from build123d import *

# Parameters (mm, degrees)
SKETCH1_W             = 15
SKETCH1_H             = 21.5
BOSS_EXTRUDE1_DEPTH   = 2.5
CHAMFER1_SIZE         = 1.5
CHAMFER1_SIZE2        = 1.7
CHAMFER1_PART_2_SIZE  = 1.5
CHAMFER1_PART_2_SIZE2 = 1.7
CHAMFER1_PART_3_SIZE  = 1.5
CHAMFER1_PART_3_SIZE2 = 1.7
CHAMFER1_PART_4_SIZE  = 1.5
CHAMFER1_PART_4_SIZE2 = 1.7
SKETCH3_W             = 11.7
SKETCH3_H             = 18
BOSS_EXTRUDE2_DEPTH   = 11
SKETCH4_W             = 6.25827791
SKETCH4_H             = 0.502489468
SKETCH4_H_2           = 0.571010759
SKETCH4_H_3           = 0.593851189
BOSS_EXTRUDE3_DEPTH   = 7
SKETCH5_R             = 0.857772401
CUT_EXTRUDE1_DEPTH    = 22
BOSS_EXTRUDE4_DEPTH   = 22
SKETCH8_W             = 6.303958771
SKETCH8_H             = 16.703004391
SKETCH8_W_2           = 12.882002706
SKETCH8_H_2           = 17.251174719
CUT_EXTRUDE2_DEPTH    = 16


with BuildPart() as part:
    # Sketch1 → Boss-Extrude1 (new body)
    with BuildSketch(Plane(origin=(0, 0, 0), x_dir=(1, 0, 0), z_dir=(0, 1, 0))):
        with Locations((1.401590457, -5.203280318)):
            Rectangle(SKETCH1_W, SKETCH1_H)
    extrude(amount=BOSS_EXTRUDE1_DEPTH)

    # Chamfer1
    chamfer1_edges = [part.edges().sort_by_distance(p)[0] for p in [
        (8.901590457, 2.5, 5.203280318),
    ]]
    chamfer1_side = [part.faces().sort_by_distance(p)[0] for p in [
        (8.901590457, 1.25, 5.203280318),
    ]]
    chamfer(chamfer1_edges, length=CHAMFER1_SIZE, length2=CHAMFER1_SIZE2, reference=chamfer1_side[0])

    # Chamfer1 part 2
    chamfer1_part_2_edges = [part.edges().sort_by_distance(p)[0] for p in [
        (1.401590457, 2.5, -5.546719682),
    ]]
    chamfer1_part_2_side = [part.faces().sort_by_distance(p)[0] for p in [
        (1.401590457, 1.25, -5.546719682),
    ]]
    chamfer(chamfer1_part_2_edges, length=CHAMFER1_PART_2_SIZE, length2=CHAMFER1_PART_2_SIZE2, reference=chamfer1_part_2_side[0])

    # Chamfer1 part 3
    chamfer1_part_3_edges = [part.edges().sort_by_distance(p)[0] for p in [
        (-6.098409543, 2.5, 5.203280318),
    ]]
    chamfer1_part_3_side = [part.faces().sort_by_distance(p)[0] for p in [
        (-6.098409543, 1.25, 5.203280318),
    ]]
    chamfer(chamfer1_part_3_edges, length=CHAMFER1_PART_3_SIZE, length2=CHAMFER1_PART_3_SIZE2, reference=chamfer1_part_3_side[0])

    # Chamfer1 part 4
    chamfer1_part_4_edges = [part.edges().sort_by_distance(p)[0] for p in [
        (1.401590457, 2.5, 15.953280318),
    ]]
    chamfer1_part_4_side = [part.faces().sort_by_distance(p)[0] for p in [
        (1.401590457, 1.25, 15.953280318),
    ]]
    chamfer(chamfer1_part_4_edges, length=CHAMFER1_PART_4_SIZE, length2=CHAMFER1_PART_4_SIZE2, reference=chamfer1_part_4_side[0])

    # Sketch3 → Boss-Extrude2 (add)
    with BuildSketch(Plane.XZ):
        with Locations((1.324498787, 5.226991199)):
            Rectangle(SKETCH3_W, SKETCH3_H)
    extrude(amount=BOSS_EXTRUDE2_DEPTH)

    # Sketch4 → Boss-Extrude3 (add)
    with BuildSketch(Plane.XZ.offset(11)):
        with Locations((1.23028723, 12.923345769)):
            Rectangle(SKETCH4_W, SKETCH4_H)
        with Locations((1.23028723, 5.854232582)):
            Rectangle(SKETCH4_W, SKETCH4_H_2)
        with Locations((1.23028723, -2.265540399)):
            Rectangle(SKETCH4_W, SKETCH4_H_3)
    extrude(amount=BOSS_EXTRUDE3_DEPTH)

    # Sketch5 → Cut-Extrude1 (cut)
    with BuildSketch(Plane(origin=(0, 0, -2.562465994), x_dir=(-1, 0, 0), z_dir=(0, 0, -1))):
        with Locations((-1.203624554, -14.610197603)):
            Circle(SKETCH5_R)
        Polygon((-3.009226286, -18.607426263), (-4.889542572, -15.232818889), (-5.175948364, -18.482902006), align=None)
        Polygon((0.726501434, -18.545164135), (2.357769206, -15.232818889), (2.818508958, -18.545164135), align=None)
    extrude(amount=-CUT_EXTRUDE1_DEPTH, mode=Mode.SUBTRACT)

    # Sketch7 → Boss-Extrude4 (add)
    with BuildSketch(Plane.ZY.offset(6.098409543)):
        with BuildLine():
            Line((12.938985356, 2.5), (-2.797520118, 2.5))
            ThreePointArc((-2.797520118, 2.5), (3.824713578, 3.86461935), (9.802054281, 7.02492997))
            ThreePointArc((9.802054281, 7.02492997), (11.710383364, 4.998077143), (12.938985356, 2.5))
        make_face()
    extrude(amount=-BOSS_EXTRUDE4_DEPTH)

    # Sketch8 → Cut-Extrude2 (cut)
    with BuildSketch(Plane(origin=(0, 2.5, 0), x_dir=(1, 0, 0), z_dir=(0, 1, 0))):
        with Locations((-6.575725783, -5.553982078)):
            Rectangle(SKETCH8_W, SKETCH8_H)
        with Locations((12.747278275, -5.828067242)):
            Rectangle(SKETCH8_W_2, SKETCH8_H_2)
    extrude(amount=CUT_EXTRUDE2_DEPTH, mode=Mode.SUBTRACT)


solid = part.part
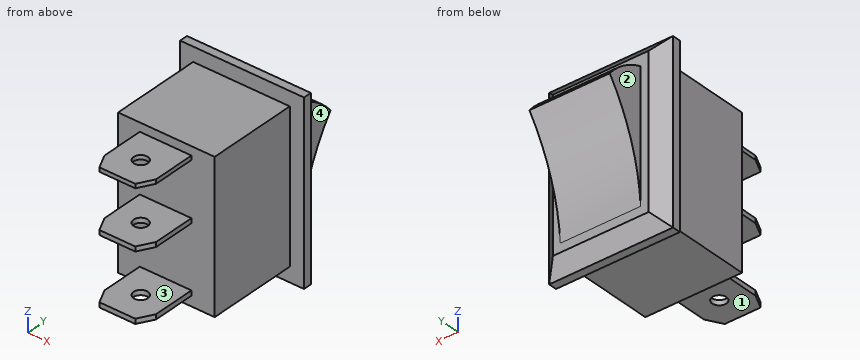
For this review, take the finished solid that the model builds, in its own axes (mm). Face numbers are marked on the shaded views. A direction names the side the tool comes from. Coordinates: 2 decimals unless noted, no trailing zeros. Loops run counter-clockwise (first coordinate to the right, second up) from the corner with the lowest first, then second, coordinate; pieces in that order, holes last. Notation, with made-up numbers: (33.5, 19) - (88.5, 19) arc R25 ccw to (88.5, 45) - close; hole circle Ø10 at (-28, -18). An arc over 180 degrees is marked (long way). Use a Markdown table: item, result. Add a question column.
Item 1: For line 1 (Z direction, x = -1.5, y = -12.5); line 2 (X direction, y = -2.5, z = 11.75); line 3 (X direction, y = 3, z = 2.5), list the stretches that pass through material, from the lowest coordinate up.
Item 2: We need section C-C (z = 12). Give the boundary of the cut face in (x, y).
Item 3: Tool access review of the marked faces 1, 2, 3 and 4: name each direction out of +Z, -Z, +X, -X, +Y, -Y from which nothing blocks a thin tool from reaching the whole face with its end or side.
Item 4: We need section B-B (x = -0.5). Give the boundary of the cut face in (y, z), and give its area (3 significant figures).
Item 5: We need section D-D (y = -16.5). Give the boundary of the cut face in (x, z).
Item 6: Insertion check: pin 1 Ø1.5 at (x, y) = (6, -4.5) entering from -Z; pin 2 Ø3.5 at (x, z) = (-1.5, 7) entering from +Y; pin 3 Ø6 at (x, z) = (-4.5, 6.5) entering from -Y; pin 4 Ø1.5 at (x, y) = (1.2, -14.61) entering from +Z. Each pin has a flat end and moves straight along its axis. Give the tip position at first contact, or say it passes through.
Item 7: We need section A-A (y = -11.75). Give the boundary of the cut face in (x, z), and give its area (3 significant figures).
Results list:
| question | item | result |
|---|---|---|
| 1 | line 1 | z = -2.56 to -1.97, 5.57 to 6.14, 12.67 to 13.17 |
| 1 | line 2 | x = -4.53 to 7.17 |
| 1 | line 3 | x = -3.42 to 6.31 |
| 2 | outline | (-6.1, 0) - (-4.53, 0) - (-4.53, -11) - (7.17, -11) - (7.17, 0) - (8.9, 0) - (8.9, 1) - (7.2, 2.5) - (6.31, 2.5) - (6.31, 4.55) - (-3.42, 4.55) - (-3.42, 2.5) - (-4.4, 2.5) - (-6.1, 1) - close |
| 3 | face 1 | -Z, +X, -X, -Y |
| 3 | face 2 | +Z, -Z, -X, +Y |
| 3 | face 3 | +X, -X, -Y |
| 3 | face 4 | +Z, -Z, +X, +Y |
| 4 | outline | (-18, -2.56) - (-11, -2.56) - (-11, -3.77) - (0, -3.77) - (0, -5.55) - (1, -5.55) - (2.5, -3.85) - (2.5, -2.8) arc R23.96 cw to (7.02, 9.8) arc R9.37 ccw to (2.5, 12.94) - (2.5, 14.25) - (1, 15.95) - (0, 15.95) - (0, 14.23) - (-11, 14.23) - (-11, 13.17) - (-18, 13.17) - (-18, 12.67) - (-11, 12.67) - (-11, 6.14) - (-18, 6.14) - (-18, 5.57) - (-11, 5.57) - (-11, -1.97) - (-18, -1.97) - close |
| 4 | area | 289 mm^2 |
| 5 | outline | (-1.73, -2.56) - (4.18, -2.56) - (4.18, -1.97) - (-1.73, -1.97) - close; (-1.73, 5.57) - (4.18, 5.57) - (4.18, 6.14) - (-1.73, 6.14) - close; (-1.73, 12.67) - (4.18, 12.67) - (4.18, 13.17) - (-1.73, 13.17) - close |
| 6 | pin 1 | stops at z = -3.77 |
| 6 | pin 2 | stops at y = 6.3 |
| 6 | pin 3 | stops at y = -16.93 |
| 6 | pin 4 | passes through |
| 7 | outline | (-1.9, -2.56) - (4.36, -2.56) - (4.36, -1.97) - (-1.9, -1.97) - close; (-1.9, 5.57) - (4.36, 5.57) - (4.36, 6.14) - (-1.9, 6.14) - close; (-1.9, 12.67) - (4.36, 12.67) - (4.36, 13.17) - (-1.9, 13.17) - close |
| 7 | area | 10.4 mm^2 |
